from build123d import *

# Parameters (mm, degrees)
BOSS_EXTRUDE1_DEPTH = 6
CUT_EXTRUDE1_REACH  = 4
SKETCH2_R           = 1.1
CUT_EXTRUDE2_REACH  = 3
SKETCH3_R           = 1.1
SKETCH5_W           = 6
SKETCH5_H           = 11
BOSS_EXTRUDE2_DEPTH = 2
CUT_EXTRUDE3_REACH  = 13
SKETCH4_R           = 0.95
CHAMFER1_SIZE       = 1


with BuildPart() as part:
    # Sketch1 → Boss-Extrude1 (new body)
    with BuildSketch(Plane.XY):
        Polygon((-1.1, 7.5), (-1.1, 0), (1.1, 0), (1.1, 7.5), (3.1, 7.5), (3.1, -3.5), (-2.1, -3.5), (-2.1, 7.5), align=None)
    extrude(amount=BOSS_EXTRUDE1_DEPTH)

    # Sketch2 → Cut-Extrude1 (cut, up to next)
    with BuildSketch(Plane.ZY.offset(-1.1), mode=Mode.PRIVATE) as cut_extrude1_sk1:
        with Locations((3, 4)):
            Circle(SKETCH2_R)
    cut_extrude1_tool1 = extrude(cut_extrude1_sk1.sketch, amount=-CUT_EXTRUDE1_REACH, mode=Mode.PRIVATE) & part.part
    add(cut_extrude1_tool1.solids().sort_by_distance((1.1, 4, 3))[0], mode=Mode.SUBTRACT)

    # Sketch3 → Cut-Extrude2 (cut, up to next)
    with BuildSketch(Plane(origin=(-1.1, 0, 0), x_dir=(0, 0, -1), z_dir=(1, 0, 0)), mode=Mode.PRIVATE) as cut_extrude2_sk1:
        with Locations((-3, 4)):
            Circle(SKETCH3_R)
    cut_extrude2_tool1 = extrude(cut_extrude2_sk1.sketch, amount=-CUT_EXTRUDE2_REACH, mode=Mode.PRIVATE) & part.part
    add(cut_extrude2_tool1.solids().sort_by_distance((-1.1, 4, 3))[0], mode=Mode.SUBTRACT)

    # Sketch5 → Boss-Extrude2 (add)
    with BuildSketch(Plane.ZY.offset(2.1)):
        with Locations((3, 2)):
            Rectangle(SKETCH5_W, SKETCH5_H)
        Polygon((5, 2.845299462), (5, 5.154700538), (3, 6.309401077), (1, 5.154700538), (1, 2.845299462), (3, 1.690598923), align=None, mode=Mode.SUBTRACT)
    extrude(amount=BOSS_EXTRUDE2_DEPTH)

    # Sketch4 → Cut-Extrude3 (cut, up to next)
    with BuildSketch(Plane.XZ.offset(3.5), mode=Mode.PRIVATE) as cut_extrude3_sk1:
        with Locations((0, 3)):
            Circle(SKETCH4_R)
    cut_extrude3_tool1 = extrude(cut_extrude3_sk1.sketch, amount=-CUT_EXTRUDE3_REACH, mode=Mode.PRIVATE) & part.part
    add(cut_extrude3_tool1.solids().sort_by_distance((0, -3.5, 3))[0], mode=Mode.SUBTRACT)

    # Chamfer1
    chamfer1_edges = [part.edges().sort_by_distance(p)[0] for p in [
        (2.1, 7.5, 0),
        (-2.6, 7.5, 6),
        (2.1, 7.5, 6),
        (-2.6, 7.5, 0),
    ]]
    chamfer(chamfer1_edges, length=CHAMFER1_SIZE)


solid = part.part
Build history of the part. All positions in model axes, mm. A direction names the side the tool comes from. Round coordinates to 2 decimals unless told otherwise and drop trailing zeros. Order: outer loops, then holes, each group sorted by start corner. A loop starts at its lowest first (then second) coordinate and runs counter-clockwise, first axis right, second up. Notation, with made-up numbers: M -14.5,47.25 L -3.5,47.25 A27 ccw -3.5,67.25 Z; hole C -24,77 d1. An arc over 180 degrees is marked long. Use CSV: the item, a comma, the result in double quotes. Start each with the question number.
(1) Drill centre lines: probe 1 along X at (y, z) = (3.5, 0.8); probe 2 along Y at (x, z) = (-1.35, 3); probe 3 along X at (y, z) = (3.5, 1.75). Where is each one in solid material? Low to high.
(2) Cut at C-C on x = -2.5. List the corners of the cut face in (y, z), then the cut area to 3 significant figures.
(3) Cut at A-A on x = 0. List the corners of the cut face in (y, z), then the cut area to 4 significant figures.
(4) Cut at B-B on y = 4. List the corners of the cut face in (x, z), then the cut area to 3 significant figures.
(5) Mould opens along X. For faces 1 (the face through (1.1, 3, 2)), 2 (the face through (-2.1, 5, 2)), 3 (the face through (2.1, 7, 0.5)) say: +X half, -X half, draft (parallel to the pull), parting line (faces both ways), or undercut.
(6) Tool access for faces 4 (the face through (-2, 1, 6)), 5 (the face through (-3.086, 2.276, 1.986)), 6 (the face through (-1.1, 3, 2)): list every direction of +Z, -Z, +X, -X, +Y, -Y with a clear straight run to the whole face (end or side of a thin tool).
(7) Cut at D-D on y = 6. List the corners of the cut face in (x, z).
Findings:
1,probe 1,"x = -4.1 to -1.1, 1.1 to 3.1"
1,probe 2,"y = -3.5 to 2.9, 5.1 to 7.5"
1,probe 3,"x = -2.1 to -1.1, 1.1 to 3.1"
2,outline,"M -3.5,0 L 6.5,0 L 7.5,1 L 7.5,5 L 6.5,6 L -3.5,6 Z; hole M 1.69,3 L 2.85,1 L 5.15,1 L 6.31,3 L 5.15,5 L 2.85,5 Z"
2,area,"51.1 mm^2"
3,outline,"M -3.5,0 L 0,0 L 0,2.05 L -3.5,2.05 Z; M -3.5,3.95 L 0,3.95 L 0,6 L -3.5,6 Z"
3,area,"14.35 mm^2"
4,outline,"M -4.1,0 L -1.1,0 L -1.1,1.9 L -2.1,1.9 L -2.1,1 L -4.1,1 Z; M -4.1,5 L -2.1,5 L -2.1,4.1 L -1.1,4.1 L -1.1,6 L -4.1,6 Z; M 1.1,0 L 3.1,0 L 3.1,1.9 L 1.1,1.9 Z; M 1.1,4.1 L 3.1,4.1 L 3.1,6 L 1.1,6 Z"
4,area,"15.4 mm^2"
5,face 1,"undercut"
5,face 2,"-X half"
5,face 3,"draft"
6,face 4,"+Z, +X, -X, +Y, -Y"
6,face 5,"-X"
6,face 6,"+Z, -Z, +Y"
7,outline,"M -4.1,0 L -1.1,0 L -1.1,6 L -4.1,6 L -4.1,3.54 L -2.1,3.54 L -2.1,2.46 L -4.1,2.46 Z; M 1.1,0 L 3.1,0 L 3.1,6 L 1.1,6 Z"
